```python
from build123d import *

# Parameters (mm, degrees)
SKETCH1_W           = 40
SKETCH1_H           = 55
BOSS_EXTRUDE1_DEPTH = 8
SKETCH1_3_W         = 40
SKETCH1_3_H         = 5
BOSS_EXTRUDE2_DEPTH = 25
SKETCH2_R           = 12
CUT_EXTRUDE1_DEPTH  = 6
CUT_EXTRUDE2_START  = -6
SKETCH2_3_R         = 10
CUT_EXTRUDE2_DEPTH  = 2


with BuildPart() as part:
    # Sketch1 → Boss-Extrude1 (new body)
    with BuildSketch(Plane(origin=(0, 0, 0), x_dir=(1, 0, 0), z_dir=(0, 1, 0))):
        with Locations((20, 27.5)):
            Rectangle(SKETCH1_W, SKETCH1_H)
    extrude(amount=BOSS_EXTRUDE1_DEPTH)

    # Sketch1<3> → Boss-Extrude2 (add)
    with BuildSketch(Plane(origin=(0, 0, 0), x_dir=(1, 0, 0), z_dir=(0, 1, 0))):
        with Locations((20, -2.5)):
            Rectangle(SKETCH1_3_W, SKETCH1_3_H)
    extrude(amount=BOSS_EXTRUDE2_DEPTH)

    # Sketch2 → Cut-Extrude1 (cut)
    with BuildSketch(Plane(origin=(0, 8, 0), x_dir=(1, 0, 0), z_dir=(0, 1, 0))):
        with Locations((20, 35)):
            Circle(SKETCH2_R)
    extrude(amount=-CUT_EXTRUDE1_DEPTH, mode=Mode.SUBTRACT)

    # Sketch2<3> → Cut-Extrude2 (cut)
    with BuildSketch(Plane(origin=(0, 8, 0), x_dir=(1, 0, 0), z_dir=(0, 1, 0)).offset(CUT_EXTRUDE2_START)):
        with Locations((20, 35)):
            Circle(SKETCH2_3_R)
    extrude(amount=-CUT_EXTRUDE2_DEPTH, mode=Mode.SUBTRACT)


solid = part.part
```
Check sheet for the modelled part. Datum: model origin and axes. Units: mm. A direction names the side the tool comes from. Round coordinates to 2 decimals unless told otherwise and drop trailing zeros. Order: outer loops, then holes, each group sorted by start corner. A loop starts at its lowest first (then second) coordinate and runs counter-clockwise, first axis right, second up.
1) Section check A-A (x = 20). Record the boundary of the cut face in (y, z), and give its area (3 significant figures).
2) Section check B-B (z = -35). Record the boundary of the cut face in (x, y), and give its area (3 significant figures).
3) Section check D-D (x = 34). Record the boundary of the cut face in (y, z), and give its area (3 significant figures).
4) Scan lines: line 1 (X direction, y = 1.55, z = -35); line 2 (Z direction, x = 20, y = 6.75); line 3 (Z direction, x = 34.5, y = 12.25). Record each from-to range of solid material in increasing order.
5) Go/stop test with flat-tipped pins: pin 1 Ø12 at (y, z) = (14.5, -28) entering from -X; pin 2 Ø12 at (x, z) = (13.5, -18.5) entering from +Y; pin 3 Ø8 at (x, z) = (5.5, -19.5) entering from -Y; pin 4 Ø1.5 at (x, y) = (24, 12.5) entering from -Z. Record where each tip stops, or that it passes through.
6) Section check C-C (y = 3.5). Record the boundary of the cut face in (x, z), and give its area (3 significant figures).
7) Tool access check on faces 4 (the cylindrical face through (8.01, 5.04, -35.53)), 5 (the flat face through (20, 8, -22)), 6 (the cylindrical face through (24.614, 1.014, -26.128)). Record the directions out of +Z, -Z, +X, -X, +Y, -Y that give a thin tool (end or side, any length) a straight path to the whole face; none if there is none.
8) Mould release check, pull along Z, two halves, no side actions. Record for faces 1 (the flat face through (15, 2, -44)), 2 (the flat face through (20, 4, -55)), 3 (the flat face through (20, 12, 5)): +Z half, -Z half, draft (parallel to the pull), parting line (faces both ways), or undercut.
Result:
1. outline: (0, -55) - (8, -55) - (8, -47) - (2, -47) - (2, -45) - (0, -45) - close; (0, -25) - (2, -25) - (2, -23) - (8, -23) - (8, 0) - (25, 0) - (25, 5) - (0, 5) - close
1. area: 381 mm2
2. outline: (0, 0) - (10, 0) - (10, 2) - (8, 2) - (8, 8) - (0, 8) - close; (30, 0) - (40, 0) - (40, 8) - (32, 8) - (32, 2) - (30, 2) - close
2. area: 136 mm2
3. outline: (0, -55) - (8, -55) - (8, 0) - (25, 0) - (25, 5) - (0, 5) - close
3. area: 565 mm2
4. line 1: x = 0 to 10, 30 to 40
4. line 2: z = -55 to -47, -23 to 5
4. line 3: z = 0 to 5
5. pin 1: passes through
5. pin 2: stops at y = 8
5. pin 3: stops at y = 0
5. pin 4: stops at z = 0
6. outline: (0, -55) - (40, -55) - (40, 5) - (0, 5) - close; hole circle Ø24 at (20, -35)
6. area: 1,950 mm2
7. face 4: +Y
7. face 5: -Z, +X, -X, +Y
7. face 6: +Y, -Y
8. face 1: undercut
8. face 2: -Z half
8. face 3: +Z half
